from build123d import *

# Parameters (mm, degrees)
EXTRUDE_1_DEPTH     = 3
SKETCH_2_R          = 1.6
SKETCH_2_R_2        = 2.1
CUT_EXTRUDE_1_DEPTH = 45.821869662
EXTRUDE_2_DEPTH     = 3


with BuildPart() as part:
    # 草图1 → 凸台-拉伸1 (new body)
    with BuildSketch(Plane.XY):
        Polygon((0, 0), (20, 0), (20, -10), (40, -10), (40, -20), (0, -20), align=None)
    extrude(amount=EXTRUDE_1_DEPTH)

    # 草图2 → 切除-拉伸1 (cut, through all)
    with BuildSketch(Plane.XY.offset(3)):
        with Locations((5, -5)):
            Circle(SKETCH_2_R)
        with Locations(Location((5, -15, 0), (0, 0, 180))):
            Circle(SKETCH_2_R)
        with Locations(Location((15, -5, 0), (0, 0, 180))):
            Circle(SKETCH_2_R)
        with Locations((15, -15)):
            Circle(SKETCH_2_R)
        with Locations((35, -15)):
            Circle(SKETCH_2_R_2)
        with Locations(Location((25, -15, 0), (0, 0, 180))):
            Circle(SKETCH_2_R_2)
    extrude(amount=-CUT_EXTRUDE_1_DEPTH, mode=Mode.SUBTRACT)

    # 草图4 → 凸台-拉伸2 (add)
    with BuildSketch(Plane.XY.offset(3)):
        Polygon((20, 0), (40, -10), (20, -10), align=None)
    extrude(amount=-EXTRUDE_2_DEPTH)


solid = part.part
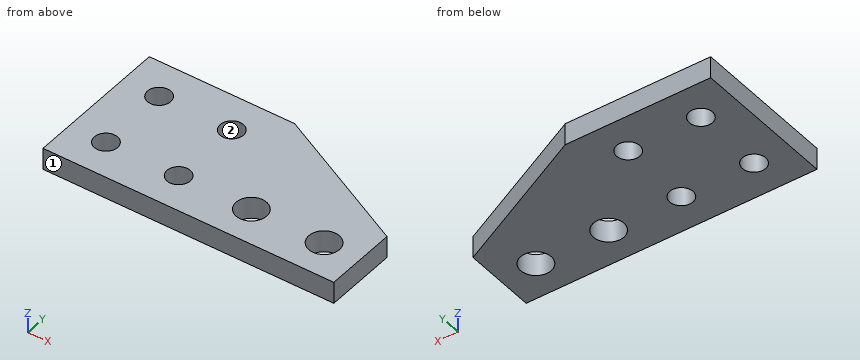
Here's how the part is built. I have some questions about the finished solid (model axes, mm). Face numbers are marked on the shaded views. Give positions to 0.01 mm unless a question says otherwise; leave off trailing zeros. Loops run counter-clockwise (first coordinate to the right, second up) from the corner with the lowest first, then second, coordinate; pieces in that order, holes last. Notation, with made-up numbers: (48.5, 87.25) -> (91.5, 87.25) arc R35 ccw to (91.5, 124.25) -> close; hole circle Ø5 at (28, -1). An arc over 180 degrees is marked (long way). One line per item, written item: value.
Q1. Suppose I cut it at D-D on x = 35. Please give me the cut outline in (y, z), then the cut area to 3 significant figures.
Answers follow:
outline: (-20, 0) -> (-17.1, 0) -> (-17.1, 3) -> (-20, 3) -> close; (-12.9, 0) -> (-7.5, 0) -> (-7.5, 3) -> (-12.9, 3) -> close
area: 24.9 mm^2
Q2. Suppose I cut it at B-B on z = 2.5. Please give me the cut outline in (x, y), then the cut area to 3 significant figures.
Answers follow:
outline: (0, -20) -> (40, -20) -> (40, -10) -> (20, 0) -> (0, 0) -> close; hole circle Ø3.2 at (5, -15); hole circle Ø3.2 at (5, -5); hole circle Ø3.2 at (15, -15); hole circle Ø3.2 at (15, -5); hole circle Ø4.2 at (25, -15); hole circle Ø4.2 at (35, -15)
area: 640 mm^2
Q3. I'm going to push a flat-ended pin straight in: pin 1 Ø2.5 at (x, y) = (5, -15) entering from +Z. Where does the tip first touch, or does it pass through?
Answers follow:
pin 1: through
Q4. Suppose I cut it at A-A on x = 15. Please give me the cut outline in (y, z), then the cut area to 3 significant figures.
Answers follow:
outline: (-20, 0) -> (-16.6, 0) -> (-16.6, 3) -> (-20, 3) -> close; (-13.4, 0) -> (-6.6, 0) -> (-6.6, 3) -> (-13.4, 3) -> close; (-3.4, 0) -> (0, 0) -> (0, 3) -> (-3.4, 3) -> close
area: 40.8 mm^2
Q5. If I drill on line 1 along Y through (x, z) = (6, 2.55); line 2 along X through (y, z) = (-14.25, 1.55); line 3 along X through (y, z) = (-16, 1.15), over which ranges is the centre line in solid material (lowest first)?
Answers follow:
line 1: -20 to -16.25, -13.75 to -6.25, -3.75 to 0
line 2: 0 to 3.59, 6.41 to 13.59, 16.41 to 23.04, 26.96 to 33.04, 36.96 to 40
line 3: 0 to 3.75, 6.25 to 13.75, 16.25 to 23.15, 26.85 to 33.15, 36.85 to 40
Q6. Suppose I cut it at C-C on y = -5. Please give me the cut outline in (x, z), then the cut area to 3 significant figures.
Answers follow:
outline: (0, 0) -> (3.4, 0) -> (3.4, 3) -> (0, 3) -> close; (6.6, 0) -> (13.4, 0) -> (13.4, 3) -> (6.6, 3) -> close; (16.6, 0) -> (30, 0) -> (30, 3) -> (16.6, 3) -> close
area: 70.8 mm^2
Q7. We'd pull the mould along X, two halves only. Please class the marked faces 1 and 2: pulls with the +X half, pulls with the -X half, needs draft (parallel to the pull), parting line crosses it, or undercut.
Answers follow:
face 1: needs draft
face 2: undercut
